Autodesk Inventor part; units mm, degrees
ref_plane "YZ Plane" through (0, 0, 0) normal (1, 0, 0) x (0, 1, 0)
ref_plane "XZ Plane" through (0, 0, 0) normal (0, 1, 0) x (-1, 0, 0)
ref_plane "XY Plane" through (0, 0, 0) normal (0, 0, 1) x (1, 0, 0)
sketch "Sketch1" plane through (0, 0, 0) normal (0, 1, 0) x (-1, 0, 0)
  line L0 (-38, 0) -> (38, 0)
  line L1 (38, 0) -> (38, 7)
  line L2 (38, 7) -> (28.5, 7)
  line L3 (28.5, 7) -> (28.5, 6)
  line L4 (28.5, 6) -> (-25.5, 6)
  line L5 (-38, 7.5926) -> (-38, 0)
  line L6 (-25.5, 6) -> (-25.5, 7.5926)
  line L7 (-25.5, 7.5926) -> (-38, 7.5926)
  point P0 (0, 0)
  point P1 (0, 0)
  dimension "d0" = 76
  dimension "d1" = 9.5
  dimension "d3" = 12.5
  dimension "d4" = 14
  dimension "d5" = 12
revolve "Revolution1" add sketch "Sketch1" angle 360 about axis through (38, 0, 0) along (-1, 0, 0)
sketch "Sketch2" plane through (0, 0, 0) normal (0, 1, 0) x (-1, 0, 0)
  line L0 (-38, -7.5926) -> (-38, 7.5926)
  line L1 (38, -7) -> (38, 7)
  line L2 (-38, 0) -> (38, 0) construction
  circle A0 centre (-30, 0) radius 2.5
  circle A1 centre (33, 0) radius 2.5
  point P0 (0, 0)
  dimension "d7" = 8
  dimension "d8" = 5
  dimension "d9" = 5
  dimension "d10" = 5
extrude "Extrusion1" cut sketch "Sketch2" against normal through all
sketch "Sketch3" plane through (38, 0, 0) normal (1, 0, 0) x (0, 0, -1)
  circle A0 centre (0, 0) radius 4
  dimension "d13" = 8
extrude "Extrusion2" add sketch "Sketch3" along normal blind 8
equation "\"d0\" = parS + stroke"
equation "\"d1\" = parNB"
equation "\"d3\" = parNA"
equation "\"d4\" = parC"
equation "\"d5\" = parB"
equation "\"d7\" = parGA"
equation "\"d8\" = parGB"
equation "\"parA\" = 15"
equation "\"parB\" = 12"
equation "\"parC\" = 14"
equation "\"parD\" = 4"
equation "\"parF\" = 8"
equation "\"parGA\" = 8"
equation "\"parGB\" = 5"
equation "\"parH\" = 28"
equation "\"parMM\" = 4"
equation "\"parNA\" = 12.5"
equation "\"parNB\" = 9.5"
equation "\"Ndh8\" = 8"
equation "\"parNN\" = 8"
equation "\"parS\" = 46"
equation "\"parZ\" = 74"
equation "\"stroke\" = 30"
properties part number "30mmCylinder"
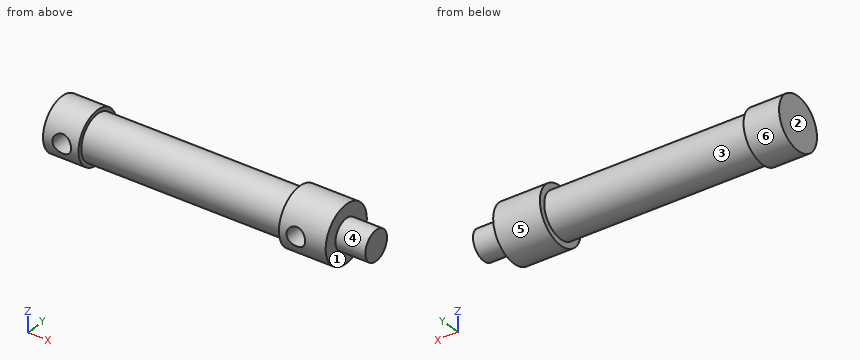
Work out the finished part from the listing and answer in its coordinate system (mm). Face numbers are marked on the shaded views. A direction names the side the tool comes from. Give positions to 0.01 mm unless a question says otherwise; leave off trailing zeros. Order: outer loops, then holes, each group sorted by start corner. A loop starts at its lowest first (then second) coordinate and runs counter-clockwise, first axis right, second up. Notation, with made-up numbers: (17, 16.25) -> (58, 16.25) arc R19 ccw to (58, 33.25) -> close; hole circle Ø9 at (-28, 63.5). An arc over 180 degrees is marked (long way). Answer as CSV lines item,"result". Start each with the question number.
(1) For a pull along X with two mould halves and no side action, classify the marked faces 1, 2, 3 and 4 as released by +X, released by -X, zero draft, split by the parting line, or undercut.
(2) Section D-D, the plane y = -5 is taken. Write down the section's boundary in (x, z), plus the area to 3 significant figures.
(3) Section C-C, the plane x = 39.5 is taken. Write down the section's boundary in (y, z), plus the area to 3 significant figures.
(4) Which of the six approach directions +Z, -Z, +X, -X, +Y, -Y give full straight-line access (tool end or side, diameter ignored) to the marked faces 5 and 6?
(5) Section B-B, the plane y = 2 is taken. Write down the section's boundary in (x, z), plus the area to 3 significant figures.
(6) Each of these flat-tipped pins is pushed along its axis until it touches: pin 1 Ø3 at (x, y) = (27, -5.5) entering from +Z; pin 2 Ø6.5 at (x, z) = (-33, 0) entering from +Y; pin 3 Ø1.5 at (y, z) = (-4.5, -4) entering from +X. Where does it stop, or does it pass through?
(7) Consider line 1 along X through (y, z) = (-5.5, 0); line 2 along X through (y, z) = (-3.25, 0); line 3 along X through (y, z) = (6, 1.5). Determine where each line is inside the solid, lowest interval first.
(8) Section A-A, the plane z = 0 is taken. Write down the section's boundary in (x, y).
Entries:
1,face 1,"released by +X"
1,face 2,"released by -X"
1,face 3,"undercut"
1,face 4,"zero draft"
2,outline,"(-38, -4.9) -> (-28.5, -4.9) -> (-28.5, -3.32) -> (25.5, -3.32) -> (25.5, -5.71) -> (38, -5.71) -> (38, 5.71) -> (25.5, 5.71) -> (25.5, 3.32) -> (-28.5, 3.32) -> (-28.5, 4.9) -> (-38, 4.9) -> close; hole circle Ø5 at (-33, 0); hole circle Ø5 at (30, 0)"
2,area,"555 mm²"
3,outline,"circle Ø8 at (0, 0)"
3,area,"50.3 mm²"
4,face 5,"+X, -X"
4,face 6,"-X"
5,outline,"(-38, -6.71) -> (-28.5, -6.71) -> (-28.5, -5.66) -> (25.5, -5.66) -> (25.5, -7.32) -> (38, -7.32) -> (38, -3.46) -> (46, -3.46) -> (46, 3.46) -> (38, 3.46) -> (38, 7.32) -> (25.5, 7.32) -> (25.5, 5.66) -> (-28.5, 5.66) -> (-28.5, 6.71) -> (-38, 6.71) -> close"
5,area,"977 mm²"
6,pin 1,"z = 6.45"
6,pin 2,"y = 7"
6,pin 3,"x = 38"
7,line 1,"-38 to -35.5, -30.5 to 27.5, 32.5 to 38"
7,line 2,"-38 to -35.5, -30.5 to 27.5, 32.5 to 46"
7,line 3,"-38 to -28.5, 25.5 to 38"
8,outline,"(-38, -7) -> (-35.5, -7) -> (-35.5, 0) -> (-30.5, 0) -> (-30.5, -7) -> (-28.5, -7) -> (-28.5, -6) -> (25.5, -6) -> (25.5, -7.59) -> (27.5, -7.59) -> (27.5, 0) -> (32.5, 0) -> (32.5, -7.59) -> (38, -7.59) -> (38, -4) -> (46, -4) -> (46, 4) -> (38, 4) -> (38, 7.59) -> (25.5, 7.59) -> (25.5, 6) -> (-28.5, 6) -> (-28.5, 7) -> (-38, 7) -> close"
